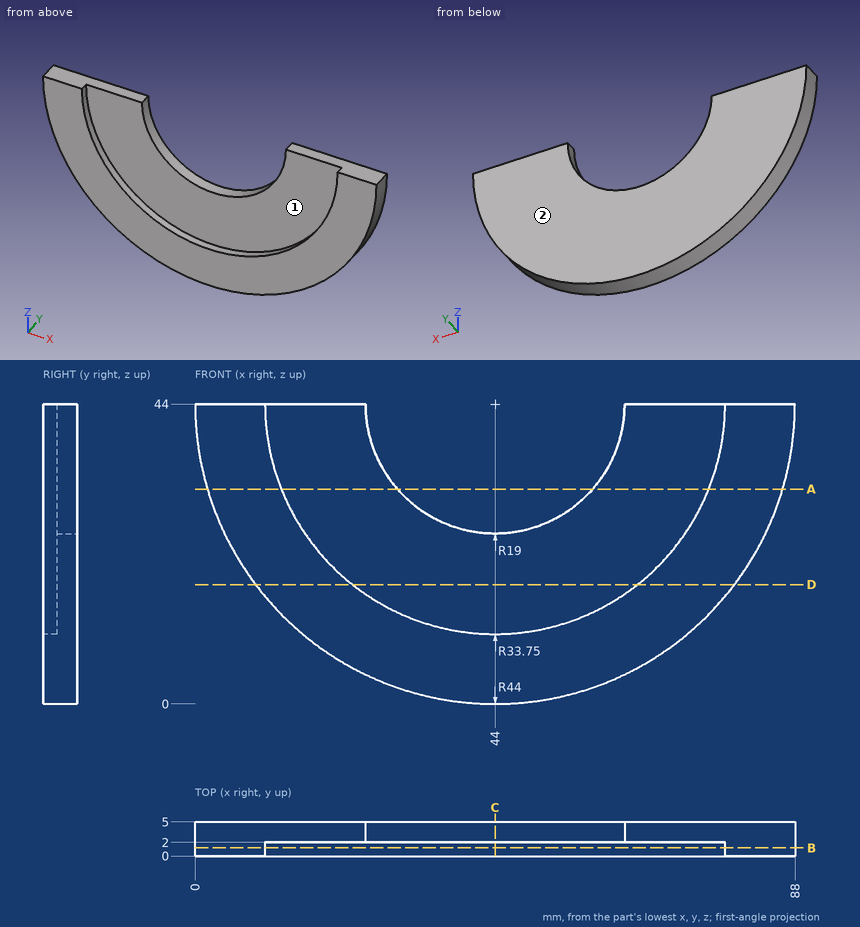
Answer from the drawing. Dimensions are ordinates in mm from the lowest x, y and z of the part. A direction names the side the tool comes from. Coordinates: 2 decimals unless noted, no trailing zeros. Write each loop counter-clockwise with the first axis right and the second up, starting at its lowest first coordinate (ties: lowest second). Pieces come first, ordered by that corner, then holes. Notation, with made-up numbers: M 81.5,1.25 L 98.5,1.25 A11 cw 98.5,17.25 Z; hole C 78,60 d2. An arc over 180 degrees is marked long. Use a Markdown table: item, result.
Q1. The part is cut by section D-D, the plane z = 17.5. Write down the section's boundary in (x, y), then the cut area to 3 significant figures.
Answer block:
| item | result |
|---|---|
| outline | M 8.88,0 L 23.1,0 L 23.1,2 L 64.9,2 L 64.9,0 L 79.12,0 L 79.12,5 L 8.88,5 Z |
| area | 268 mm2 |
Q2. Straight lines are drawn through the part: L1, parallel to X at y = 0.6, z = 31; L2, parallel to X at y = 0.6, z = 27; L3, parallel to Z at x = 44, y = 1.45. For each, find the intervals that lie inside material, in ascending order. Write a range as [from, to].
Answer block:
| item | result |
|---|---|
| L1 | x = [1.96, 12.85], [75.15, 86.04] |
| L2 | x = [3.42, 14.84], [73.16, 84.58] |
| L3 | z = [0, 10.25] |
Q3. The part is cut by section B-B, the plane y = 1.2. Write down the section's boundary in (x, z).
Answer block:
| item | result |
|---|---|
| outline | M 0,44 A44 ccw 88,44 L 77.75,44 A33.75 cw 10.25,44 Z |
Q4. Each of these flat-tipped pins is pushed along its axis until it touches: pin 1 Ø3 at (x, z) = (51, 30) entering from +Y; pin 2 Ø2 at (y, z) = (2.5, 12) entering from +X (3 decimals); pin 3 Ø3 at (x, y) = (29, 3.5) entering from +Z; pin 4 Ø3 at (x, y) = (21.5, 3.5) entering from -Z. Where does it stop, or does it pass through?
Answer block:
| item | result |
|---|---|
| pin 1 | passes through |
| pin 2 | stops at x = 75.225 |
| pin 3 | stops at z = 34.58 |
| pin 4 | stops at z = 5.33 |
Q5. The part is cut by section A-A, the plane z = 31.5. Write down the section's boundary in (x, y).
Answer block:
| item | result |
|---|---|
| outline | M 1.81,0 L 12.65,0 L 12.65,2 L 29.69,2 L 29.69,5 L 1.81,5 Z; M 58.31,2 L 75.35,2 L 75.35,0 L 86.19,0 L 86.19,5 L 58.31,5 Z |
Q6. The part is cut by section C-C, the plane x = 44. Write down the section's boundary in (y, z), then the cut area to 3 significant figures.
Answer block:
| item | result |
|---|---|
| outline | M 0,0 L 5,0 L 5,25 L 2,25 L 2,10.25 L 0,10.25 Z |
| area | 95.5 mm2 |
Q7. Which of the six approach directions +Z, -Z, +X, -X, +Y, -Y give full straight-line access (tool end or side, diameter ignored) to the marked faces 1 and 2?
Answer block:
| item | result |
|---|---|
| face 1 | +Z, -Y |
| face 2 | +Z, -Z, +X, -X, +Y |
